```python
from build123d import *

# Parameters (mm, degrees)
SKETCH3_R          = 1.2
CUT_EXTRUDE1_DEPTH = 24
SKETCH4_W          = 2
SKETCH4_H          = 8
CUT_EXTRUDE2_DEPTH = 4
CHAMFER1_SIZE      = 1
CUT_EXTRUDE3_START = -21.7
CUT_EXTRUDE3_DEPTH = 21.7


with BuildPart() as part:
    # Sketch2 → Revolve1 (revolve)
    with BuildSketch(Plane(origin=(0, 0, 0), x_dir=(1, 0, 0), z_dir=(0, 1, 0)), mode=Mode.PRIVATE) as revolve1_sk:
        Polygon((0, 0), (0, 3), (24, 3), (24, 6), (30, 6), (30, 0), align=None)
    revolve(revolve1_sk.sketch.rotate(Axis((0, 0, 0), (1, 0, 0)), 180), axis=Axis((0, 0, 0), (1, 0, 0)))

    # Sketch3 → Cut-Extrude1 (cut)
    with BuildSketch(Plane.ZY):
        Circle(SKETCH3_R)
    extrude(amount=-CUT_EXTRUDE1_DEPTH, mode=Mode.SUBTRACT)

    # Sketch4 → Cut-Extrude2 (cut)
    with BuildSketch(Plane(origin=(30, 0, 0), x_dir=(0, 0, -1), z_dir=(1, 0, 0))):
        Rectangle(SKETCH4_W, SKETCH4_H)
    extrude(amount=-CUT_EXTRUDE2_DEPTH, mode=Mode.SUBTRACT)

    # Chamfer1
    chamfer1_edges = [part.edges().sort_by_distance(p)[0] for p in [
        (30, 0, -6),
        (24, 0, -6),
    ]]
    chamfer(chamfer1_edges, length=CHAMFER1_SIZE)

    # Sketch5 → Cut-Extrude3 (cut)
    with BuildSketch(Plane.ZY.offset(CUT_EXTRUDE3_START)):
        with BuildLine():
            Line((-0.9, 2.861817604), (-0.9, 1.78605711))
            ThreePointArc((-0.9, 1.78605711), (0, 2), (0.9, 1.78605711))
            Line((0.9, 1.78605711), (0.9, 2.861817604))
            ThreePointArc((0.9, 2.861817604), (0, 3), (-0.9, 2.861817604))
        make_face()
        with BuildLine():
            Line((-0.9, -1.78605711), (-0.9, -2.861817604))
            ThreePointArc((-0.9, -2.861817604), (0, -3), (0.9, -2.861817604))
            Line((0.9, -2.861817604), (0.9, -1.78605711))
            ThreePointArc((0.9, -1.78605711), (0, -2), (-0.9, -1.78605711))
        make_face()
    extrude(amount=CUT_EXTRUDE3_DEPTH, mode=Mode.SUBTRACT)


solid = part.part
```
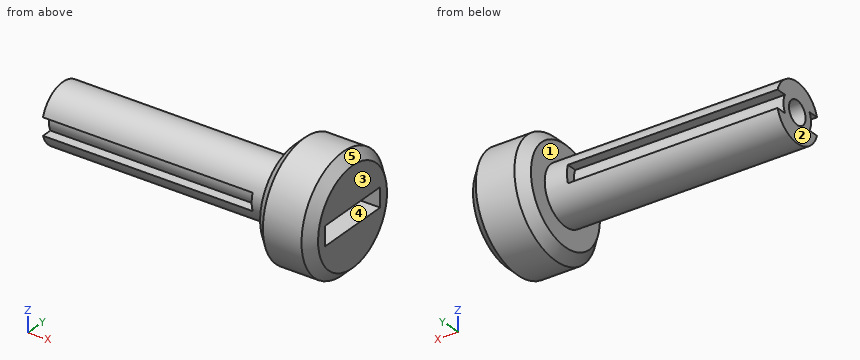
Design review of the part built by this model. Coordinates are the model's own, in mm. Face numbers are marked on the shaded views. A direction names the side the tool comes from. Coordinates: 2 decimals unless noted, no trailing zeros. Loops run counter-clockwise (first coordinate to the right, second up) from the corner with the lowest first, then second, coordinate; pieces in that order, holes last. Notation, with made-up numbers: M 32.25,36 L 86.25,36 A29 cw 86.25,70 Z; hole C 37.25,59.25 d10. An arc over 180 degrees is marked long. One line per question, with ' | ' between items.
(1) We need section B-B (z = 0). Give the boundary of the cut face in (x, y).
Filled in:
outline: M 0,-2 L 21.7,-2 L 21.7,-3 L 24,-3 L 24,-5 L 25,-6 L 29,-6 L 30,-5 L 30,-4 L 26,-4 L 26,4 L 30,4 L 30,5 L 29,6 L 25,6 L 24,5 L 24,3 L 21.7,3 L 21.7,2 L 0,2 L 0,1.2 L 24,1.2 L 24,-1.2 L 0,-1.2 Z
(2) Machinability: for the marked faces 1 and 2, which of the approach directions +Z, -Z, +X, -X, +Y, -Y give a long, thin tool a straight path to every point of the face, cutting with its end or side? Answer none if there is none.
Filled in:
face 1: -X | face 2: +Z, -Z, -X, +Y, -Y
(3) We need section C-C (x = 24.5). Give the boundary of the cut face in (y, z), and give its area (3 significant figures).
Filled in:
outline: C 0,0 d11 | area: 95.0 mm^2
(4) Wall thickness on probe 1 along Z at (x, y) = (10.5, -2.75); probe 2 along X at (y, z) = (0.75, -0.75); probe 3 along X at (y, z) = (2.75, -2.5): over which ranges is each line inside the solid? List them lowest first.
Filled in:
probe 1: z = -1.2 to -0.9, 0.9 to 1.2 | probe 2: x = 24 to 26 | probe 3: x = 24 to 30
(5) For pin 1 Ø0.9 at (x, y) = (12, 2) entering from -Z; pin 2 Ø1.5 at (y, z) = (4, 0.5) entering from -X; pin 3 Ø1 at (y, z) = (-3, 0) entering from -X, all flat-tipped, find the tip position at first contact; note any pin that passes through.
Filled in:
pin 1: stops at z = -2.57 | pin 2: stops at x = 24 | pin 3: stops at x = 21.7
(6) We need section D-D (x = 28). Give the boundary of the cut face in (y, z).
Filled in:
outline: C 0,0 d12; hole M -4,-1 L 4,-1 L 4,1 L -4,1 Z
(7) We need section A-A (x = 9.25). Give the boundary of the cut face in (y, z).
Filled in:
outline: M -2.86,-0.9 A3 ccw 2.86,-0.9 L 1.79,-0.9 A2 ccw 1.79,0.9 L 2.86,0.9 A3 ccw -2.86,0.9 L -1.79,0.9 A2 ccw -1.79,-0.9 Z; hole C 0,0 d2.4
(8) Draft analysis for pull direction Y (two halves, no side actions). For the marked faces 3, 4 and 5, state which applies: released by +Y, released by -Y, zero draft, split by the parting line, or undercut.
Filled in:
face 3: zero draft | face 4: undercut | face 5: split by the parting line
